from build123d import *

# Parameters (mm, degrees)
F0_W           = 20
F0_H           = 15
F1_DEPTH       = 2
F3_D           = 3.3
F3_CSINK_D     = 6.72
F3_CSINK_ANGLE = 90
F4_R           = 1.5
F5_DEPTH       = 2.001
F6_R           = 2


with BuildPart() as f1:
    # F0 (on Front) → F1 (new body)
    with BuildSketch(Plane.XZ):
        with Locations((10, 7.5)):
            Rectangle(F0_W, F0_H)
    extrude(amount=-F1_DEPTH)

    # F3 (through all)
    with Locations(Plane.XZ):
        with Locations((15.5, 10.5), (4.5, 4.5)):
            CounterSinkHole(F3_D / 2, F3_CSINK_D / 2, counter_sink_angle=F3_CSINK_ANGLE)

    # F4 (on face) → F5 (cut, through all)
    with BuildSketch(Plane.XZ):
        with Locations((15.5, 4.5)):
            Circle(F4_R)
        with Locations((4.5, 10.5)):
            Circle(F4_R)
    extrude(amount=-F5_DEPTH, mode=Mode.SUBTRACT)

    # F6
    f6_edges = [f1.edges().sort_by_distance(p)[0] for p in [
        (20, 1, 15),
        (0, 1, 15),
        (20, 1, 0),
        (0, 1, 0),
    ]]
    fillet(f6_edges, radius=F6_R)


solid = f1.part
Work out the finished part from the listing and answer in its coordinate system (mm). Coordinates: 2 decimals unless noted, no trailing zeros. Write each loop counter-clockwise with the first axis right and the second up, starting at its lowest first coordinate (ties: lowest second). Pieces come first, ordered by that corner, then holes.
1. The part is cut by section B-B, the plane y = 1.2. Write down the section's boundary in (x, z).
Results list:
outline: (0, 2) arc R2 ccw to (2, 0) - (18, 0) arc R2 ccw to (20, 2) - (20, 13) arc R2 ccw to (18, 15) - (2, 15) arc R2 ccw to (0, 13) - close; hole circle Ø4.32 at (4.5, 4.5); hole circle Ø3 at (4.5, 10.5); hole circle Ø4.32 at (15.5, 10.5); hole circle Ø3 at (15.5, 4.5)
2. Flat-ended cylindrical pins translate along their axes: pin 1 (2 mm diameter, centred on x = 4, z = 6, fed in from -Y); pin 2 (2 mm diameter, centred on x = 15.5, z = 10.5, fed in from -Y). Find the tip coordinate at first contact, or state that the pin passes through.
Results list:
pin 1: stops at y = 0.78
pin 2: passes through
3. For a pull along X with two mould halves and no side action, classify faces 1 (the flat face through (0, 1, 7)), 2 (the cylindrical face through (14, 0.99, 4.57)), 3 (the cylindrical face through (19.4, 1.01, 0.57)), 4 (the flat face through (10, 0, 8)) as +X half, -X half, draft (parallel to the pull), parting line (faces both ways), or undercut.
Results list:
face 1: -X half
face 2: undercut
face 3: +X half
face 4: draft
4. The part is cut by section A-A, the plane z = 4.5. Write down the section's boundary in (x, y), and give its area (3 significant figures).
Results list:
outline: (0, 0) - (1.14, 0) - (2.85, 1.71) - (2.85, 2) - (0, 2) - close; (6.15, 1.71) - (7.86, 0) - (14, 0) - (14, 2) - (6.15, 2) - close; (17, 0) - (20, 0) - (20, 2) - (17, 2) - close
area: 24.5 mm2
5. The part is cut by section D-D, the plane y = 0.3. Write down the section's boundary in (x, z), and give its area (3 significant figures).
Results list:
outline: (0, 2) arc R2 ccw to (2, 0) - (18, 0) arc R2 ccw to (20, 2) - (20, 13) arc R2 ccw to (18, 15) - (2, 15) arc R2 ccw to (0, 13) - close; hole circle Ø6.12 at (4.5, 4.5); hole circle Ø3 at (4.5, 10.5); hole circle Ø6.12 at (15.5, 10.5); hole circle Ø3 at (15.5, 4.5)
area: 224 mm2
6. The part is cut by section C-C, the plane x = 15.5. Write down the section's boundary in (y, z).
Results list:
outline: (0, 0) - (2, 0) - (2, 3) - (0, 3) - close; (0, 6) - (2, 6) - (2, 8.85) - (1.71, 8.85) - (0, 7.14) - close; (0, 13.86) - (1.71, 12.15) - (2, 12.15) - (2, 15) - (0, 15) - close
7. Consider line 1 along Z through (x, y) = (15.5, 1.95); line 2 along Z through (x, y) = (4.5, 1.8); line 3 along X through (y, z) = (1.3, 4). Determine where each line is inside the solid, lowest interval first.
Results list:
line 1: z = 0 to 3, 6 to 8.85, 12.15 to 15
line 2: z = 0 to 2.85, 6.15 to 9, 12 to 15
line 3: x = 0 to 2.5, 6.5 to 14.09, 16.91 to 20
